```python
from build123d import *

# Parameters (mm, degrees)
BOSS_EXTRUDE1_DEPTH = 5
SKETCH2_R           = 1.625
CUT_EXTRUDE1_DEPTH  = 5
SKETCH3_W           = 7
SKETCH3_H           = 3
CUT_EXTRUDE2_DEPTH  = 5
SKETCH4_R           = 1.375
BOSS_EXTRUDE2_DEPTH = 3
CUT_EXTRUDE3_DEPTH  = 5
FILLET1_R           = 2
FILLET2_R           = 4
FILLET3_R           = 40
FILLET5_R           = 2
FILLET6_R           = 2
FILLET7_R           = 3
FILLET10_R          = 1.5


# Some blends are built 0.0001 mm under size
with BuildPart() as part:
    # Sketch1 → Boss-Extrude1 (new body)
    with BuildSketch(Plane(origin=(0, 0, 0), x_dir=(1, 0, 0), z_dir=(0, 1, 0))):
        with BuildLine():
            Line((0, 145), (0, 85))
            ThreePointArc((0, 85), (1.979630786, 42.309847603), (8, 0))
            Line((8, 0), (24, 0))
            ThreePointArc((24, 0), (28.920632518, 43.079645644), (40, 85))
            Line((40, 85), (40, 100))
            Line((40, 100), (15, 100))
            Line((15, 100), (15, 140))
            Line((15, 140), (40, 140))
            Line((40, 140), (40, 145))
            ThreePointArc((40, 145), (20, 150), (0, 145))
        make_face()
    extrude(amount=BOSS_EXTRUDE1_DEPTH)

    # Sketch2 → Cut-Extrude1 (cut)
    with BuildSketch(Plane(origin=(0, 5, 0), x_dir=(1, 0, 0), z_dir=(0, 1, 0))):
        with Locations(Location((7.5, 131, 0), (0, 0, 270))):
            Circle(SKETCH2_R)
        with Locations(Location((7.5, 115, 0), (0, 0, 270))):
            Circle(SKETCH2_R)
    extrude(amount=-CUT_EXTRUDE1_DEPTH, mode=Mode.SUBTRACT)

    # Sketch3 → Cut-Extrude2 (cut)
    with BuildSketch(Plane(origin=(0, 5, 0), x_dir=(1, 0, 0), z_dir=(0, 1, 0))):
        with Locations((27.5, 98.5)):
            Rectangle(SKETCH3_W, SKETCH3_H)
    extrude(amount=-CUT_EXTRUDE2_DEPTH, mode=Mode.SUBTRACT)

    # Sketch4 → Boss-Extrude2 (add)
    with BuildSketch(Plane(origin=(0, 0, -97), x_dir=(-1, 0, 0), z_dir=(0, 0, -1))):
        with Locations(Location((-27.5, 2.5, 0), (0, 0, 180))):
            Circle(SKETCH4_R)
    extrude(amount=BOSS_EXTRUDE2_DEPTH)

    # Sketch5 → Cut-Extrude3 (cut)
    with BuildSketch(Plane(origin=(0, 5, 0), x_dir=(1, 0, 0), z_dir=(0, 1, 0))):
        with BuildLine():
            Line((14, 90), (30, 90))
            Line((30, 90), (30, 87))
            Line((30, 87), (30, 86.654767806))
            ThreePointArc((30, 86.654767806), (20.590082312, 52.378278053), (15.165707783, 17.249935341))
            ThreePointArc((15.165707783, 17.249935341), (11.273342316, 51.022188328), (10, 84.994150003))
            Line((10, 84.994150003), (10, 90))
            Line((10, 90), (14, 90))
        make_face()
    extrude(amount=-CUT_EXTRUDE3_DEPTH, mode=Mode.SUBTRACT)

    # Fillet1
    fillet1_edges = [part.edges().sort_by_distance(p)[0] for p in [
        (10, 2.5, -90),
        (30, 2.5, -90),
    ]]
    fillet(fillet1_edges, radius=FILLET1_R)

    # Fillet2
    fillet2_edges = [part.edges().sort_by_distance(p)[0] for p in [
        (30, 2.5, -86.654767806),
    ]]
    fillet(fillet2_edges, radius=FILLET2_R)

    # Fillet3
    fillet3_edges = [part.edges().sort_by_distance(p)[0] for p in [
        (40, 2.5, -85),
    ]]
    fillet(fillet3_edges, radius=FILLET3_R)

    # Fillet5
    fillet5_edges = [part.edges().sort_by_distance(p)[0] for p in [
        (15, 2.5, -140),
        (15, 2.5, -100),
    ]]
    fillet(fillet5_edges, radius=FILLET5_R)

    # Fillet6
    fillet6_edges = [part.edges().sort_by_distance(p)[0] for p in [
        (40, 2.5, -140),
        (40, 2.5, -100),
    ]]
    fillet(fillet6_edges, radius=FILLET6_R)

    # Fillet7
    fillet7_edges = [part.edges().sort_by_distance(p)[0] for p in [
        (40, 2.5, -145),
        (0, 2.5, -145),
    ]]
    fillet(fillet7_edges, radius=FILLET7_R)

    # Fillet8
    # a fillet whose section is not a circle: 2 mm, written as the material it adds along each edge
    with BuildSketch(Plane(origin=(15.165707783, 5, -17.249935341), x_dir=(0.12048141281398392, 0, -0.9927155832192553), z_dir=(0, -1, 0))) as fillet8_piece_1:
        with BuildLine():
            Bezier((15.455336501, 0), (0.383468278, -0.375827748), (15.032037076, -3.942603658), weights=[1, 1, 1])
            ThreePointArc((15.032037076, -3.942603658), (7.498610953, -2.037672046), (0, 0))
            ThreePointArc((0, 0), (7.72766825, -0.096332478), (15.455336501, 0))
        make_face()
    extrude(amount=5)

    # Fillet10
    fillet10_edges = [part.edges().sort_by_distance(p)[0] for p in [
        (31, 2.5, -97),
        (24, 2.5, -97),
    ]]
    fillet(fillet10_edges, radius=FILLET10_R)
    fillet10_2_edges = [part.edges().sort_by_distance(p)[0] for p in [
        (31, 2.5, -100),
        (24, 2.5, -100),
    ]]
    fillet(fillet10_2_edges, radius=FILLET10_R - 0.0001)  # a hair under: the kernel refuses the full size


solid = part.part
```
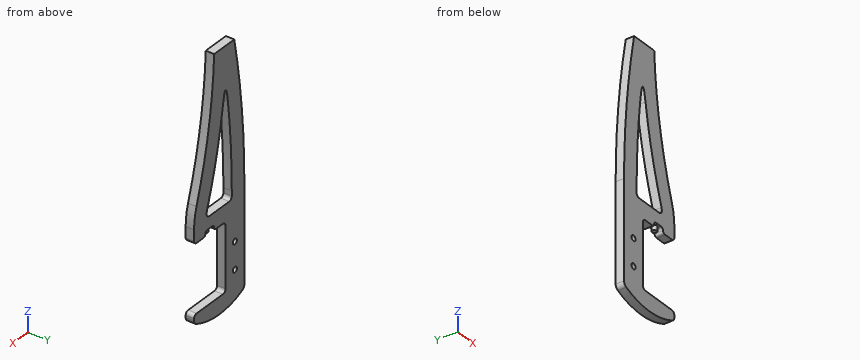
For this review, take the finished solid that the model builds, in its own axes (mm). Give positions to 0.01 mm unless a question says otherwise; leave off trailing zeros. Loops run counter-clockwise (first coordinate to the right, second up) from the corner with the lowest first, then second, coordinate; pieces in that order, holes last. Notation, with made-up numbers: M 15.25,-31.5 L 59.25,-31.5 A30 cw 59.25,-7.5 Z; hole C 29.25,-34 d6. An arc over 180 degrees is marked long. One line per item, written item: value. Start each with the question number.
Q1. For L1, parallel to X at y = 2.4, z = -131 (3 decimals); L2, parallel to X at y = 2.25, z = -122; L3, parallel to Z at x = 15.5, y = 1.25, list the stretches that pass through material, from the lowest coordinate up.
Q2. Add section A-A (z = -131). Give the boundary of the cut face in (x, y) (3 decimals).
Q3. Clearance check with flat-ended pins moving along their axes: pin 1 Ø1.5 at (x, y) = (36.5, 2.5) entering from -Z; pin 2 Ø2.5 at (y, z) = (1.5, -86) entering from +X; pin 3 Ø1.5 at (y, z) = (2, -17) entering from -X. State where each tip first meets the part, or that it passes through.
Q4. Add section B-B (y = 2.5). Count the separate pieces of the cut face and the enclosed holes in it, and give its area (3 significant figures).
Q5. Add section C-C (z = -45.5). Give the boundary of the cut face in (x, y).
Reply:
1. L1: 0 to 5.875, 9.125 to 15
1. L2: 0 to 15
1. L3: -149.76 to -139.32, -100.68 to -90, -25.72 to 0
2. outline: M 0,0 L 5.875,0 L 5.875,5 L 0,5 Z; M 9.125,0 L 15,0 L 15,5 L 9.125,5 Z
3. pin 1: z = -146.97
3. pin 2: x = 39.78
3. pin 3: x = 4.97
4. separate pieces: 1
4. enclosed holes: 3
4. area: 3,100 mm²
5. outline: M 1.69,0 L 11.73,0 L 11.73,5 L 1.69,5 Z; M 19.2,0 L 29.39,0 L 29.39,5 L 19.2,5 Z
